```python
from build123d import *

# Parameters (mm, degrees)
SKETCH_1_R      = 1.25
EXTRUDE_1_DEPTH = 1.15
FILLET_1_R      = 0.2


with BuildPart() as part:
    # 草图1 → 凸台-拉伸1 (new body, symmetric)
    with BuildSketch(Plane(origin=(0, 0, 0), x_dir=(1, 0, 0), z_dir=(0, 1, 0))):
        Polygon((2.886751346, 0), (1.443375673, 2.5), (-1.443375673, 2.5), (-2.886751346, 0), (-1.443375673, -2.5), (1.443375673, -2.5), align=None)
        Circle(SKETCH_1_R, mode=Mode.SUBTRACT)
    extrude(amount=EXTRUDE_1_DEPTH, both=True)

    # 草图2 → 切除-旋转1 (revolve, cut)
    with BuildSketch(Plane.XY):
        Polygon((-2.886751346, 0.85), (-2.3, 1.15), (-2.886751346, 1.15), align=None)
    cut_revolve_1 = revolve(axis=Axis((0, 1.15, 0), (0, -1, 0)), mode=Mode.SUBTRACT)

    # 镜向1: 切除-旋转1 across plane
    add(cut_revolve_1.mirror(Plane.ZX), mode=Mode.SUBTRACT)

    # 草图3 → 旋转1 (revolve)
    with BuildSketch(Plane(origin=(0, 0, 0), x_dir=(0, 0, -1), z_dir=(1, 0, 0))):
        with BuildLine():
            Line((-2.3, 1.15), (-2.3, 1.55))
            ThreePointArc((-2.3, 1.55), (-1.796008242, 1.773528846), (-1.25, 1.85))
            Line((-1.25, 1.85), (-1.25, 1.15))
            Line((-1.25, 1.15), (-2.3, 1.15))
        make_face()
    revolve(axis=Axis((0, 1.15, 0), (0, -1, 0)))

    # 圆角1
    fillet_1_edges = [part.edges().sort_by_distance(p)[0] for p in [
        (1.626345597, 1.15, -1.626345597),
        (0, 1.55, -2.3),
        (0, 1.85, -1.25),
    ]]
    fillet(fillet_1_edges, radius=FILLET_1_R)


solid = part.part
```
The model under review builds one solid part; all positions refer to its coordinate system, in mm. Round coordinates to 2 decimals unless told otherwise and drop trailing zeros. Write each loop counter-clockwise with the first axis right and the second up, starting at its lowest first coordinate (ties: lowest second). Pieces come first, ordered by that corner, then holes.
(1) We need section A-A on y = -0.2. Give the boundary of the cut face in (x, z).
(2) Mouldability with a two-part tool opening along Y and no side actions: class faces 1 (the flat face through (1, -1.15, 1)), 2 (the flat face through (-2.155, 0.015, -1.268)) as +Y half, -Y half, draft (parallel to the pull), parting line (faces both ways), or undercut.
(3) Wall thickness on L1, parallel to Z at x = 0, y = 0.4; L2, parallel to Z at x = 0, y = 1.35; L3, parallel to X at y = 0.4, z = 0.8: over which ranges is each line inside the solid? List them lowest first.
Findings below:
1. outline: (-2.89, 0) - (-1.44, -2.5) - (1.44, -2.5) - (2.89, 0) - (1.44, 2.5) - (-1.44, 2.5) - close; hole circle Ø2.5 at (0, 0)
2. face 1: -Y half
2. face 2: draft
3. L1: z = -2.5 to -1.25, 1.25 to 2.5
3. L2: z = -2.3 to -1.25, 1.25 to 2.3
3. L3: x = -2.42 to -0.96, 0.96 to 2.42
